from build123d import *

# Parameters (mm, degrees)
SKETCH2_W           = 60
SKETCH2_H           = 30
BOSS_EXTRUDE1_DEPTH = 28
BOSS_EXTRUDE3_DEPTH = 20
SKETCH6_R           = 6
CUT_EXTRUDE7_DEPTH  = 60


with BuildPart() as part:
    # Sketch2 → Boss-Extrude1 (new body)
    with BuildSketch(Plane(origin=(0, 0, 0), x_dir=(1, 0, 0), z_dir=(0, 1, 0))):
        with Locations((30, 15)):
            Rectangle(SKETCH2_W, SKETCH2_H)
    extrude(amount=BOSS_EXTRUDE1_DEPTH)

    # Sketch3 → Boss-Extrude3 (add)
    with BuildSketch(Plane.XY):
        Polygon((0, 28), (0, 73), (20, 73), (20, 48), (32, 48), (32, 36), (48, 36), (48, 28), align=None)
    extrude(amount=-BOSS_EXTRUDE3_DEPTH)

    # Sketch6 → Cut-Extrude7 (cut)
    with BuildSketch(Plane(origin=(0, 0, -30), x_dir=(-1, 0, 0), z_dir=(0, 0, -1))):
        with Locations((-44, 16)):
            Circle(SKETCH6_R)
    extrude(amount=-CUT_EXTRUDE7_DEPTH, mode=Mode.SUBTRACT)


solid = part.part
Can you work these out from the model? Positions are in its coordinate system, mm. A direction names the side the tool comes from. Give positions to 0.01 mm unless a question says otherwise; leave off trailing zeros. Loops run counter-clockwise (first coordinate to the right, second up) from the corner with the lowest first, then second, coordinate; pieces in that order, holes last. Notation, with made-up numbers: M 59,-7 L 109,-7 A7 ccw 109,1 Z; hole C 44.5,52.25 d2. An arc over 180 degrees is marked long. One line per item, written item: value.
1) I'm going to push flat-ended pins straight in: pin 1 (2 mm diameter, centred on y = 50, z = -8, fed in from +X); pin 2 (9.5 mm diameter, centred on x = 25, z = -13.5, fed in from +Y); pin 3 (4 mm diameter, centred on y = 31, z = -9, fed in from +X). Where does each tip first touch, or does it pass through?
Geometry check:
pin 1: stops at x = 20
pin 2: stops at y = 48
pin 3: stops at x = 48
2) Imagine slicing it at B-B on z = -9. Write out the boundary of the cut face in (x, y).
Geometry check:
outline: M 0,0 L 60,0 L 60,28 L 48,28 L 48,36 L 32,36 L 32,48 L 20,48 L 20,73 L 0,73 Z; hole C 44,16 d12
3) Imagine slicing it at D-D on x = 16. Write out the boundary of the cut face in (y, z), and give its area (3 significant figures).
Geometry check:
outline: M 0,-30 L 28,-30 L 28,-20 L 73,-20 L 73,0 L 0,0 Z
area: 1,740 mm²
4) On a 3-axis mill with a long thin cutter (end or side, diameter ignored), from which of +Z, -Z, +X, -X, +Y, -Y can I reach the whole of each face in a straight line? I mean faces 1 (the face through (19, 46, -20)), 2 (the face through (40, 36, -10)), 3 (the face through (10, 73, -10)). Say none if no direction works.
Geometry check:
face 1: -Z, +X, -X, +Y
face 2: +Z, -Z, +X, +Y
face 3: +Z, -Z, +X, -X, +Y
5) Imagine slicing it at A-A on x = 44. Write out the boundary of the cut face in (y, z), and give its area (3 significant figures).
Geometry check:
outline: M 0,-30 L 10,-30 L 10,0 L 0,0 Z; M 22,-30 L 28,-30 L 28,-20 L 36,-20 L 36,0 L 22,0 Z
area: 640 mm²
6) Imagine slicing it at C-C on y = 16. Write out the boundary of the cut face in (x, z), and give its area (3 significant figures).
Geometry check:
outline: M 0,-30 L 38,-30 L 38,0 L 0,0 Z; M 50,-30 L 60,-30 L 60,0 L 50,0 Z
area: 1,440 mm²
7) Thinking about a two-plate mould opening in X: for faces 4 (the face through (48, 32, -10)), 5 (the face through (50, 16, -15)), 6 (the face through (24, 29, 0)), which applies, +X half, -X half, draft (parallel to the pull), parting line (faces both ways), or undercut?
Geometry check:
face 4: +X half
face 5: undercut
face 6: draft
8) Please list where these lines run through material, in increasing order: line 1 (Y direction, x = 44, z = -8); line 2 (X direction, y = 57.5, z = -6); line 3 (Y direction, x = 16, z = -25.5).
Geometry check:
line 1: y = 0 to 10, 22 to 36
line 2: x = 0 to 20
line 3: y = 0 to 28
